Verification items for the finished model (mm, model axes). Face numbers are marked on the shaded views. A direction names the side the tool comes from. Round coordinates to 2 decimals unless told otherwise and drop trailing zeros. Write each loop counter-clockwise with the first axis right and the second up, starting at its lowest first coordinate (ties: lowest second). Pieces come first, ordered by that corner, then holes. Notation, with made-up numbers: (55.5, -1.75) -> (97.5, -1.75) arc R28 ccw to (97.5, 21.25) -> close; hole circle Ø5 at (-7.5, 80.5). An arc over 180 degrees is marked (long way). Answer as a JSON object with one key per item and string values. Group by question number.
(1) Sectioned sample at C-C on z = 4.5. Record the cut outline in (x, y).
(2) Scan lines: L1, parallel to X at y = 1.25, z = 0; L2, parallel to Y at x = 4.5, z = 2.5; L3, parallel to Y at x = 2.5, z = -0.5. Record each from-to range of solid material in increasing order. Write a range as from..to.
(3) Sectioned sample at D-D on y = -2. Record the cut outline in (x, z), and give its area (3 significant figures).
(4) Sectioned sample at A-A on y = -28. Record the cut outline in (x, z).
(5) Gauge pin test, flat ends, axial feed: pin 1 Ø0.5 at (x, y) = (-8, -31.5) entering from -Z; pin 2 Ø4.5 at (x, y) = (-0.5, -29.5) entering from +Z; pin 3 Ø6 at (y, z) = (-21.5, -7.5) entering from -X. Record the tip position at first contact, or that the pin passes through.
(6) Sectioned sample at B-B on y = -20.5. Record the cut outline in (x, z), and give its area (3 significant figures).
(7) Set-up check for the marked faces 1, 2, 3, 4 and 5: record each of +Z, -Z, +X, -X, +Y, -Y from which the full face is reachable in a straight line by a thin tool's end or side.
(8) Draft check along Z on the marked faces 6, 7 and 8. Enter one of: released by +Z, released by -Z, zero draft, split by the parting line, or undercut.
```python
from build123d import *

# Parameters (mm, degrees)
ESQUISSE1_R             = 11
BOSS_EXTRU_1_DEPTH      = 14.5
ESQUISSE2_R             = 12.35
BOSS_EXTRU_2_DEPTH      = 2
ESQUISSE3_R             = 9
ENL_V_MAT_EXTRU_1_DEPTH = 1
ESQUISSE4_R             = 10.5
BOSS_EXTRU_3_DEPTH      = 12.5
ESQUISSE5_W             = 1
ESQUISSE5_H             = 4
ESQUISSE5_W_2           = 4
ESQUISSE5_H_2           = 1
BOSS_EXTRU_4_DEPTH      = 6
BOSS_EXTRU_5_START      = 6
BOSS_EXTRU_5_DEPTH      = 2


with BuildPart() as part:
    # Esquisse1 → Boss.-Extru.1 (new body)
    with BuildSketch(Plane(origin=(0, 0, 0), x_dir=(1, 0, 0), z_dir=(0, 1, 0))):
        with Locations(Location((0, 0, 0), (0, 0, 270))):
            Circle(ESQUISSE1_R)
    extrude(amount=-BOSS_EXTRU_1_DEPTH)

    # Esquisse2 → Boss.-Extru.2 (add)
    with BuildSketch(Plane(origin=(0, 0, 0), x_dir=(1, 0, 0), z_dir=(0, 1, 0))):
        with Locations(Location((0, 0, 0), (0, 0, 270))):
            Circle(ESQUISSE2_R)
    extrude(amount=BOSS_EXTRU_2_DEPTH)

    # Esquisse3 → Enlèv. mat.-Extru.1 (cut)
    with BuildSketch(Plane(origin=(0, 2, 0), x_dir=(1, 0, 0), z_dir=(0, 1, 0))):
        with Locations(Location((0, 0, 0), (0, 0, 270))):
            Circle(ESQUISSE3_R)
        with BuildLine():
            Line((-1, 0), (-1, 6.394930003))
            ThreePointArc((-1, 6.394930003), (0, 7.394930003), (1, 6.394930003))
            Line((1, 6.394930003), (1, 0))
            ThreePointArc((1, 0), (0, -1), (-1, 0))
        make_face(mode=Mode.SUBTRACT)
        with BuildLine():
            ThreePointArc((-3.641353304, 4.768704868), (0, -6), (3.641353304, 4.768704868))
            ThreePointArc((3.641353304, 4.768704868), (2.239676942, 4.58081294), (2.427568869, 3.179136578))
            ThreePointArc((2.427568869, 3.179136578), (0, -4), (-2.427568869, 3.179136578))
            ThreePointArc((-2.427568869, 3.179136578), (-2.239676942, 4.58081294), (-3.641353304, 4.768704868))
        make_face(mode=Mode.SUBTRACT)
    extrude(amount=-ENL_V_MAT_EXTRU_1_DEPTH, mode=Mode.SUBTRACT)

    # Esquisse4 → Boss.-Extru.3 (add)
    with BuildSketch(Plane.XZ.offset(14.5)):
        with Locations(Location((0, 0, 0), (0, 0, 270))):
            Circle(ESQUISSE4_R)
    extrude(amount=BOSS_EXTRU_3_DEPTH)

    # Esquisse5 → Boss.-Extru.4 (add)
    with BuildSketch(Plane.XZ.offset(27)):
        with Locations((-8, 0)):
            Rectangle(ESQUISSE5_W, ESQUISSE5_H)
        with Locations((0, 8)):
            Rectangle(ESQUISSE5_W_2, ESQUISSE5_H_2)
        with Locations((0, -8)):
            Rectangle(ESQUISSE5_W_2, ESQUISSE5_H_2)
        with Locations((8, 0)):
            Rectangle(ESQUISSE5_W, ESQUISSE5_H)
    extrude(amount=BOSS_EXTRU_4_DEPTH)

    # Esquisse6 → Boss.-Extru.5 (add)
    with BuildSketch(Plane.XZ.offset(BOSS_EXTRU_5_START)):
        Polygon((14, 0), (7, 12.124355653), (-7, 12.124355653), (-14, 0), (-7, -12.124355653), (7, -12.124355653), align=None)
    extrude(amount=BOSS_EXTRU_5_DEPTH)


solid = part.part
```
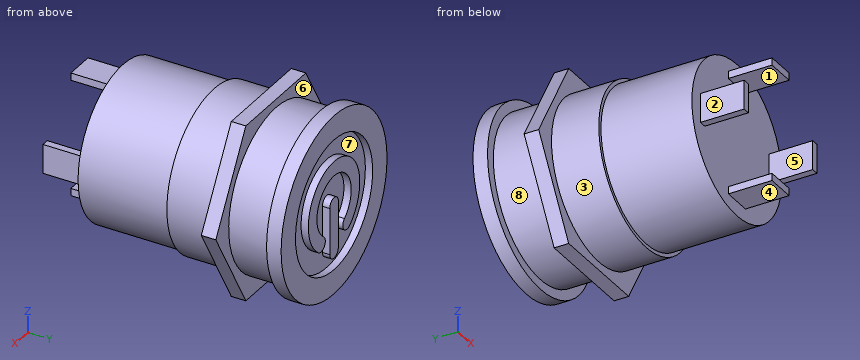
Computed values:
{
 "1": {"outline": "(-11.5, 0) -> (-10.04, 0) -> (-10.04, -6) -> (-11.4, -6) -> (-11.4, -8) -> (-10.04, -8) -> (-10.04, -14.5) -> (-9.49, -14.5) -> (-9.49, -27) -> (9.49, -27) -> (9.49, -14.5) -> (10.04, -14.5) -> (10.04, -8) -> (11.4, -8) -> (11.4, -6) -> (10.04, -6) -> (10.04, 0) -> (11.5, 0) -> (11.5, 2) -> (7.79, 2) -> (7.79, 1) -> (3.97, 1) -> (3.97, 2) -> (-3.97, 2) -> (-3.97, 1) -> (-7.79, 1) -> (-7.79, 2) -> (-11.5, 2) -> close"},
 "2": {"L1": "-12.35..-9, -6..-4, -1..1, 4..6, 9..12.35", "L2": "-27..2", "L3": "-27..1"},
 "3": {"outline": "circle Ø22 at (0, 0)", "area": "380 mm2"},
 "4": {"outline": "(-8.5, -2) -> (-7.5, -2) -> (-7.5, 2) -> (-8.5, 2) -> close; (-2, -8.5) -> (2, -8.5) -> (2, -7.5) -> (-2, -7.5) -> close; (-2, 7.5) -> (2, 7.5) -> (2, 8.5) -> (-2, 8.5) -> close; (7.5, -2) -> (8.5, -2) -> (8.5, 2) -> (7.5, 2) -> close"},
 "5": {"pin 1": "z = -2", "pin 2": "z = 8.5", "pin 3": "x = -9.49"},
 "6": {"outline": "circle Ø21 at (0, 0)", "area": "346 mm2"},
 "7": {"face 1": "+X, -X, -Y", "face 2": "+Z, -Z, -X, -Y", "face 3": "-Y", "face 4": "-Z, +X, -X, -Y", "face 5": "+Z, -Z, -Y"},
 "8": {"face 6": "zero draft", "face 7": "undercut", "face 8": "split by the parting line"}
}
